Check sheet for the modelled part. Datum: model origin and axes. Units: mm. A direction names the side the tool comes from. Coordinates: 2 decimals unless noted, no trailing zeros. Write each loop counter-clockwise with the first axis right and the second up, starting at its lowest first coordinate (ties: lowest second). Pieces come first, ordered by that corner, then holes. Notation, with made-up numbers: (79.25, 88.25) -> (89.25, 88.25) arc R26 cw to (89.25, 127.25) -> close; hole circle Ø11 at (-21.5, -30). An arc over 180 degrees is marked (long way). Put each result on its own line as item: value.
```python
from build123d import *

# Parameters (mm, degrees)
F1_DEPTH = 100
F2_SIZE  = 4
F3_SIZE  = 6
F4_R     = 1.9
F5_DEPTH = 8
F6_R     = 4
F7_DEPTH = 2.5


with BuildPart() as f1:
    # F0 (on Top) → F1 (new body)
    with BuildSketch(Plane.XY):
        Polygon((-14.065653, 8.299918), (-34.065653, 8.299918), (-34.065653, 1.799918), (1.434347, 1.799918), (1.434347, 11.799918), (-6.565653, 11.799918), (-6.565653, 14.299918), (1.434347, 14.299918), (1.434347, 18.299918), (-14.065653, 18.299918), align=None)
    extrude(amount=F1_DEPTH)

    # F2
    f2_edges = [f1.edges().sort_by_distance(p)[0] for p in [
        (-16.315653, 1.799918, 100),
        (-16.315653, 1.799918, 0),
        (1.434347, 1.799918, 50),
    ]]
    chamfer(f2_edges, length=F2_SIZE)

    # F3
    f3_edges = [f1.edges().sort_by_distance(p)[0] for p in [
        (-34.065653, 1.799918, 50),
    ]]
    chamfer(f3_edges, length=F3_SIZE)

    # F4 (on face) → F5 (cut)
    with BuildSketch(Plane.XZ.offset(-1.799918)):
        with Locations((-23.065653, 90)):
            Circle(F4_R)
        with Locations((-23.065653, 10)):
            Circle(F4_R)
    extrude(amount=-F5_DEPTH, mode=Mode.SUBTRACT)

    # F6 (on face) → F7 (cut)
    with BuildSketch(Plane.XZ.offset(-1.799918)):
        with Locations((-23.065653, 90)):
            Circle(F6_R)
        with Locations((-23.065653, 10)):
            Circle(F6_R)
    extrude(amount=-F7_DEPTH, mode=Mode.SUBTRACT)


solid = f1.part
```
Q1. Cross-section at B-B (z = 77). Record the cut outline in (x, y), plus the area to 3 significant figures.
Recorded:
outline: (-34.07, 7.8) -> (-28.07, 1.8) -> (-2.57, 1.8) -> (1.43, 5.8) -> (1.43, 11.8) -> (-6.57, 11.8) -> (-6.57, 14.3) -> (1.43, 14.3) -> (1.43, 18.3) -> (-14.07, 18.3) -> (-14.07, 8.3) -> (-34.07, 8.3) -> close
area: 340 mm2
Q2. Cross-section at C-C (y = 16). Record the cut outline in (x, z), plus the area to 3 significant figures.
Recorded:
outline: (-14.07, 0) -> (1.43, 0) -> (1.43, 100) -> (-14.07, 100) -> close
area: 1,550 mm2
Q3. Cross-section at D-D (x = -31). Record the cut outline in (y, z).
Recorded:
outline: (4.73, 1.07) -> (5.8, 0) -> (8.3, 0) -> (8.3, 100) -> (5.8, 100) -> (4.73, 98.93) -> close
Q4. Mould release check, pull along Z, two halves, no side actions. Record for faces 6 (the flat face through (-15.6, 3.8, 98)), 7 (the cylindrical face through (-22.189, 6.272, 88.314)), 8 (the flat face through (-3, 14.3, 49)): released by +Z, released by -Z, zero draft, split by the parting line, or undercut.
Recorded:
face 6: released by +Z
face 7: undercut
face 8: zero draft
Q5. Depth check by flat-ended pin: P1, Ø10, axis at x = -25.5, z = 40, coming from the +Y side; P2, Ø7, axis at x = -23.07, z = 90, coming from the -Y side; P3, Ø0.8, axis at y = 13, z = 68.5, coming from the +X side. Enter the tip coordinate at first touch or a pass-through.
Recorded:
P1: stops at y = 8.3
P2: stops at y = 4.3
P3: stops at x = -6.57
Q6. Cross-section at A-A (z = 90). Record the cut outline in (x, y), plus the area to 3 significant figures.
Recorded:
outline: (-34.07, 7.8) -> (-28.07, 1.8) -> (-27.07, 1.8) -> (-27.07, 4.3) -> (-24.97, 4.3) -> (-24.97, 8.3) -> (-34.07, 8.3) -> close; (-21.17, 4.3) -> (-19.07, 4.3) -> (-19.07, 1.8) -> (-2.57, 1.8) -> (1.43, 5.8) -> (1.43, 11.8) -> (-6.57, 11.8) -> (-6.57, 14.3) -> (1.43, 14.3) -> (1.43, 18.3) -> (-14.07, 18.3) -> (-14.07, 8.3) -> (-21.17, 8.3) -> close
area: 305 mm2
Q7. Material ranges on line 1 along Y through (x, z) = (-3, 54); line 2 along X through (y, z) = (11.25, 35.5); line 3 along Y through (x, z) = (-24, 75), recorded low to high.
Recorded:
line 1: y = 1.8 to 11.8, 14.3 to 18.3
line 2: x = -14.07 to 1.43
line 3: y = 1.8 to 8.3
Q8. Tool access check on faces 1 (the flat face through (-14.066, 13, 49)), 2 (the flat face through (1.434, 9, 49)), 3 (the flat face through (-6.566, 13, 49)), 4 (the cylindrical face through (-19.25, 3.03, 11.2)), 5 (the flat face through (-0.538, 3.828, 49.3)). Record the directions out of +Z, -Z, +X, -X, +Y, -Y that give a thin tool (end or side, any length) a straight path to the whole face; none if there is none.
Recorded:
face 1: +Z, -Z, -X, +Y
face 2: +Z, -Z, +X, +Y, -Y
face 3: +Z, -Z, +X
face 4: -Y
face 5: +Z, -Z, +X, -Y
